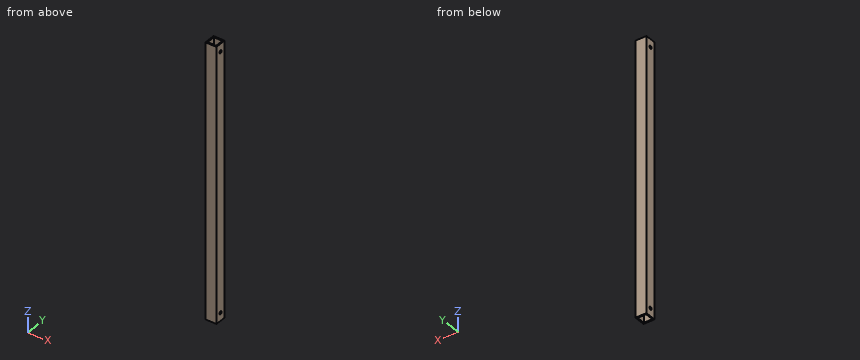
```python
from build123d import *

# Parameters (mm, degrees)
SKETCH_1_W             = 25
SKETCH_1_H             = 25
SKETCH_1_W_2           = 19
SKETCH_1_H_2           = 19
EXTRUDE_1_DEPTH        = 616
HOLE_WIZARD_7_0_7_1_D  = 7
PATTERN_LINEAR_1_COUNT = 2
PATTERN_LINEAR_1_PITCH = 580.3


with BuildPart() as part:
    # 草图1 → 拉伸1 (new body)
    with BuildSketch(Plane.XY):
        with Locations((12.5, -12.5)):
            Rectangle(SKETCH_1_W, SKETCH_1_H)
        with Locations((12.5, -12.5)):
            Rectangle(SKETCH_1_W_2, SKETCH_1_H_2, mode=Mode.SUBTRACT)
    extrude(amount=EXTRUDE_1_DEPTH)

    # Ø7.0 (7) 直径孔1 (through all)
    with Locations(Plane(origin=(25, 0, 0), x_dir=(0, 0, -1), z_dir=(1, 0, 0))):
        with Locations((-598.15, -12.5)):
            hole_wizard_7_0_7_1 = Hole(HOLE_WIZARD_7_0_7_1_D / 2)

    # 阵列(线性)1: Ø7.0 (7) 直径孔1 ×2
    with Locations(*[(0, 0, -i * PATTERN_LINEAR_1_PITCH) for i in range(1, PATTERN_LINEAR_1_COUNT)]):
        add(hole_wizard_7_0_7_1, mode=Mode.SUBTRACT)


solid = part.part
```
Here's how the part is built. I have some questions about the finished solid (model axes, mm). Coordinates: 2 decimals unless noted, no trailing zeros. Loops run counter-clockwise (first coordinate to the right, second up) from the corner with the lowest first, then second, coordinate; pieces in that order, holes last. Notation, with made-up numbers: (19.5, 54.25) - (31.5, 54.25) arc R19 cw to (31.5, 81.25) - close; hole circle Ø6 at (-10.5, -23.75). An arc over 180 degrees is marked (long way). Answer as CSV lines item,"result".
Q1. If we section it at B-B, the plane z = 134: Write out the boundary of the cut face in (x, y), and give its area (3 significant figures).
Response:
outline,"(0, -25) - (25, -25) - (25, 0) - (0, 0) - close; hole (3, -22) - (22, -22) - (22, -3) - (3, -3) - close"
area,"264 mm2"
Q2. For pin 1 (5.5 mm diameter, centred on y = -12.5, z = 598.15, fed in from +X); pin 2 (8 mm diameter, centred on y = -12.5, z = 17.85, fed in from +X), each with a flat end and sliding along its axis, tell me the tip position at first contact or that it passes through.
Response:
pin 1,"through"
pin 2,"x = 25"
Q3. If we section it at A-A, the plane x = 17.75: Write out the boundary of the cut face in (y, z), and give its area (3 significant figures).
Response:
outline,"(-25, 0) - (-22, 0) - (-22, 616) - (-25, 616) - close; (-3, 0) - (0, 0) - (0, 616) - (-3, 616) - close"
area,"3,700 mm2"
Q4. If I drill on L1, parallel to X at y = -15.25, z = 454; L2, parallel to Y at x = 4.5, z = 446; L3, parallel to Y at x = 23.4, z = 17.85, over which ranges is the centre line in solid material (lowest first)? Write a range as [from, to].
Response:
L1,"[0, 3], [22, 25]"
L2,"[-25, -22], [-3, 0]"
L3,"[-25, -16], [-9, 0]"
